CAD build for the part. Positions are in the model's coordinates, mm. A direction names the side the tool comes from. Round coordinates to 2 decimals unless told otherwise and drop trailing zeros. Loops run counter-clockwise (first coordinate to the right, second up) from the corner with the lowest first, then second, coordinate; pieces in that order, holes last. Notation, with made-up numbers: M -39,42.25 L -2,42.25 A22 ccw -2,67.25 Z; hole C 22,30.5 d2. An arc over 180 degrees is marked long. Put each result on its own line as item: value. Start each with the question number.
Solid Edge part; units mm, degrees
sketch "Sketch1" plane through (0, 0, 0) normal (0, -1, 0) x (1, 0, 0)
  line L0 (-32, 46) -> (-65.7571, 46)
  line L1 (0, 0) -> (0, 30)
  arc A0 (0, 30) -> (-32, 46) centre (0, 70) cw
  arc A1 (0, 0) -> (-65.7571, 46) centre (0, 70) cw
extrude "Protrusion1" add sketch "Sketch1" along normal mid plane 10
sketch "Sketch2" plane through (-32.8786, -5, 23) normal (0, -1, 0) x (1, 0, 0)
  line L0 (-7.1214, 47) -> (-37.1214, 47)
  line L1 (32.8786, -23) -> (32.8786, 7)
  arc A0 (32.8786, 7) -> (-7.1214, 47) centre (32.8786, 47) cw
  arc A1 (32.8786, -23) -> (-37.1214, 47) centre (32.8786, 47) cw
extrude "ExtrudedProtrusion_2" add sketch "Sketch2" along normal blind 10
sketch "Sketch3" plane through (-32.8786, 5, 23) normal (0, 1, 0) x (-1, 0, 0)
  line L0 (-32.8786, -23) -> (-32.8786, 7)
  line L1 (37.1214, 47) -> (7.1214, 47)
  arc A0 (37.1214, 47) -> (-32.8786, -23) centre (-32.8786, 47) cw
  arc A1 (7.1214, 47) -> (-32.8786, 7) centre (-32.8786, 47) cw
extrude "ExtrudedProtrusion_3" add sketch "Sketch3" along normal blind 10
sketch "Sketch4" plane through (0, 0, 0) normal (0, 0, 1) x (1, 0, 0)
  line L0 (-8.5091, 47.5) -> (-8.5091, -47.5)
  arc A0 (-8.5091, 47.5) -> (-8.5091, -47.5) centre (7.1034, 0) cw
extrude "ExtrudedProtrusion_4" add sketch "Sketch4" along normal blind 25
sketch "Sketch5" plane through (24.2972, 0, 25) normal (0, 0, 1) x (0, 1, 0)
  line L0 (0, -14.8062) -> (15, -14.8062)
  line L1 (15, -14.8062) -> (15, -32.8062)
  line L2 (15, -32.8062) -> (-15, -32.8062)
  line L3 (-15, -32.8062) -> (-15, -14.8062)
  line L4 (-15, -14.8062) -> (0, -14.8062)
extrude "ExtrudedCutout_2" cut sketch "Sketch5" against normal blind 5
(1) Cut at C-C on x = -3.5. List the corners of the cut face in (y, z), and give its area (3 significant figures).
(2) Cut at D-D on z = 14. List the corners of the cut face in (x, y), and give its area (3 significant figures).
(3) Mould opens along Y. For faces 1 (the cylindrical face through (57.086, 1.322, 12.325)), 2 (the flat face through (39.103, 0, 23)), 3 (the flat face through (-55, -10, 70)) say: +Y half, -Y half, draft (parallel to the pull), parting line (faces both ways), or undercut.
(4) Cut at B-B on y = 0. List the corners of the cut face in (x, z), and give its area (3 significant figures).
(5) Drill centre lines: line 1 along Z through (x, y) = (38.5, 13); line 2 along Y through (x, z) = (-22, 30); line 3 along Z through (x, y) = (41.5, 14). Where is each one in solid material? Low to high.
(6) Flat gauge pins, fed straight in: pin 1 Ø1.5 at (x, y) = (10.5, 26) entering from +Z; pin 2 Ø5.5 at (x, z) = (47.5, 22.5) entering from +Y; pin 3 Ø3 at (x, y) = (-50.5, 1) entering from +Z. Where does each tip first touch, or does it go through?
(7) Tool access for faces 4 (the flat face through (47, 15, 23)), 5 (the flat face through (0, 0, 27)), 6 (the flat face through (17, 1, 0)), 7 (the flat face through (-55, 5, 58)): list every direction of +Z, -Z, +X, -X, +Y, -Y with a clear straight run to the whole face (end or side of a thin tool).
(8) Cut at A-A on z = 61. List the corners of the cut face in (x, y), and give its area (3 significant figures).
Taken from the geometry:
1. outline: M -48.86,0 L 48.86,0 L 48.86,25 L 15,25 L 15,30.15 L -15,30.15 L -15,25 L -48.86,25 Z
1. area: 2,600 mm2
2. outline: M -42,-15 L -8.51,-15 L -8.51,-47.5 A50 ccw long -8.51,47.5 L -8.51,15 L -42,15 Z
2. area: 6,470 mm2
3. face 1: parting line
3. face 2: undercut
3. face 3: draft
4. outline: M -65.76,46 A70 ccw -8.51,0.52 L -8.51,0 L 57.1,0 L 57.1,20 L 39.1,20 L 39.1,25 L 0,25 L 0,30 A40 cw -32,46 Z
4. area: 3,180 mm2
5. line 1: 0 to 25
5. line 2: -15 to 15
5. line 3: 0 to 20
6. pin 1: z = 25
6. pin 2: y = 32.9
6. pin 3: z = 46
7. face 4: +Z, +X
7. face 5: +Z, +X, +Y, -Y
7. face 6: -Z, +X, -X, +Y, -Y
7. face 7: +Z, +X, -X
8. outline: M -69.42,-15 L -38.97,-15 L -38.97,-5 L -69.42,-5 Z; M -69.42,5 L -38.97,5 L -38.97,15 L -69.42,15 Z
8. area: 609 mm2
